For this review, take the finished solid that the model builds, in its own axes (mm). A direction names the side the tool comes from. Coordinates: 2 decimals unless noted, no trailing zeros. Write each loop counter-clockwise with the first axis right and the second up, starting at its lowest first coordinate (ties: lowest second). Pieces come first, ordered by that corner, then holes. Notation, with made-up numbers: (9, -26) -> (34, -26) arc R18 ccw to (34, -1) -> close; hole circle Ø7 at (53, -21.75). An arc over 180 degrees is marked (long way). Put each result on its own line as item: value. Start each with the question number.
Item 1: The part is to be moulded in two halves that separate along X. For faces 1 (the flat face through (72, 39, 4.762)), 2 (the cylindrical face through (79.41, 64.095, 2.348)), 3 (the flat face through (0.794, 38, 2)), say which applies: +X half, -X half, draft (parallel to the pull), parting line (faces both ways), or undercut.
Item 2: To check wall thickness, follow L1, parallel to Y at x = 113.5, z = 0.25; L2, parallel to Y at x = 72.39, z = 3.8; L3, parallel to X at y = 30, z = 3.95. State the ranges of each line that lie inside material, in increasing order.
Item 3: Consider section D-D on x = 120. Give the boundary of the cut face in (y, z).
Item 4: For faces 4 (the flat face through (4, 55.562, 2)), 5 (the flat face through (11.24, 8, 2)), 6 (the flat face through (142, 55.562, 2)), 7 (the cylindrical face through (122.29, 60.74, 2.35)), 8 (the flat face through (134.81, 8, 2)), list the 3-axis set-ups (+Z, -Z, +X, -X, +Y, -Y) from which the entire face can be reached by the end or side of a thin tool; tool diameter is ignored.
Item 5: Consider section C-C on z = 4. Give the number of separate pieces and of enclosed holes in the cut face, and give its area (3 significant figures).
Item 6: Consider section A-A on y = 45.72. Give the boundary of the cut face in (x, z).
Item 7: Consider section B-B on x = 72.39. Give the boundary of the cut face in (y, z), and give its area (3 significant figures).
Item 8: Insertion check: P1, Ø15, axis at x = 72.39, y = 57.658, coming from the -Z side; P2, Ø1.5, axis at x = 103.5, y = 54.5, coming from the -Z side; P3, Ø2, axis at x = 142.5, z = 1.5, coming from the +Y side; P4, Ø1.4, axis at y = 65.5, z = 1.5, coming from the +X side. Each pin has a flat end and moves straight along its axis. Give the tip position at first contact, or say it passes through.
```python
from build123d import *

# Parameters (mm, degrees)
BOSS_EXTRUDE1_DEPTH         = 4.7625
F_3_4_0_75_DIAMETER_HOLE1_D = 19.05
F_6_CLEARANCE_HOLE1_D       = 4.3053


with BuildPart() as part:
    # Sketch1 → Boss-Extrude1 (new body)
    with BuildSketch(Plane.XY):
        with BuildLine():
            Line((134.8105, 61.9125), (134.8105, 73.88225))
            ThreePointArc((134.8105, 73.88225), (134.364130735, 74.959880735), (133.2865, 75.40625))
            Line((133.2865, 75.40625), (12.7635, 75.40625))
            ThreePointArc((12.7635, 75.40625), (11.685869265, 74.959880735), (11.2395, 73.88225))
            Line((11.2395, 73.88225), (11.2395, 61.9125))
            ThreePointArc((11.2395, 61.9125), (9.379628061, 57.422371939), (4.8895, 55.5625))
            Line((4.8895, 55.5625), (2.31775, 55.5625))
            ThreePointArc((2.31775, 55.5625), (1.240119265, 55.116130735), (0.79375, 54.0385))
            Line((0.79375, 54.0385), (0.79375, 22.1615))
            ThreePointArc((0.79375, 22.1615), (1.240119265, 21.083869265), (2.31775, 20.6375))
            Line((2.31775, 20.6375), (4.8895, 20.6375))
            ThreePointArc((4.8895, 20.6375), (9.379628061, 18.777628061), (11.2395, 14.2875))
            Line((11.2395, 14.2875), (11.2395, 2.31775))
            ThreePointArc((11.2395, 2.31775), (11.685869265, 1.240119265), (12.7635, 0.79375))
            Line((12.7635, 0.79375), (133.2865, 0.79375))
            ThreePointArc((133.2865, 0.79375), (134.364130735, 1.240119265), (134.8105, 2.31775))
            Line((134.8105, 2.31775), (134.8105, 14.2875))
            ThreePointArc((134.8105, 14.2875), (136.670371939, 18.777628061), (141.1605, 20.6375))
            Line((141.1605, 20.6375), (143.73225, 20.6375))
            ThreePointArc((143.73225, 20.6375), (144.809880735, 21.083869265), (145.25625, 22.1615))
            Line((145.25625, 22.1615), (145.25625, 54.0385))
            ThreePointArc((145.25625, 54.0385), (144.809880735, 55.116130735), (143.73225, 55.5625))
            Line((143.73225, 55.5625), (141.1605, 55.5625))
            ThreePointArc((141.1605, 55.5625), (136.670371939, 57.422371939), (134.8105, 61.9125))
        make_face()
    extrude(amount=BOSS_EXTRUDE1_DEPTH)

    # 3/4 (0.75) Diameter Hole1 (through all)
    with Locations(Plane.XY.offset(4.7625)):
        with Locations((31.75, 60.325), (72.39, 57.658), (112.776, 60.325), (112.776, 22.225), (38.1, 22.225)):
            Hole(F_3_4_0_75_DIAMETER_HOLE1_D / 2)

    # #6 Clearance Hole1 (through all)
    with Locations(Plane.XY.offset(4.7625)):
        with Locations((18.034, 45.72), (128.016, 45.72)):
            Hole(F_6_CLEARANCE_HOLE1_D / 2)


solid = part.part
```
Return value:
1. face 1: draft
1. face 2: undercut
1. face 3: -X half
2. L1: 0.79 to 12.73, 31.72 to 50.83, 69.82 to 75.41
2. L2: 0.79 to 48.13, 67.18 to 75.41
2. L3: 0.79 to 32.6, 43.6 to 107.27, 118.28 to 145.26
3. outline: (0.79, 0) -> (16.02, 0) -> (16.02, 4.76) -> (0.79, 4.76) -> close; (28.43, 0) -> (54.12, 0) -> (54.12, 4.76) -> (28.43, 4.76) -> close; (66.53, 0) -> (75.41, 0) -> (75.41, 4.76) -> (66.53, 4.76) -> close
4. face 4: +Z, -Z, -X, +Y
4. face 5: +Z, -Z, -X, -Y
4. face 6: +Z, -Z, +X, +Y
4. face 7: +Z, -Z
4. face 8: +Z, -Z, +X, -Y
5. separate pieces: 1
5. enclosed holes: 7
5. area: 8,530 mm^2
6. outline: (0.79, 0) -> (15.88, 0) -> (15.88, 4.76) -> (0.79, 4.76) -> close; (20.19, 0) -> (125.86, 0) -> (125.86, 4.76) -> (20.19, 4.76) -> close; (130.17, 0) -> (145.26, 0) -> (145.26, 4.76) -> (130.17, 4.76) -> close
7. outline: (0.79, 0) -> (48.13, 0) -> (48.13, 4.76) -> (0.79, 4.76) -> close; (67.18, 0) -> (75.41, 0) -> (75.41, 4.76) -> (67.18, 4.76) -> close
7. area: 265 mm^2
8. P1: through
8. P2: z = 0
8. P3: y = 55.56
8. P4: x = 134.81
